Can you work these out from the model? Positions are in its coordinate system, mm. A direction names the side the tool comes from. Give positions to 0.01 mm unless a question says otherwise; leave off trailing zeros. Write each loop counter-clockwise with the first axis right and the second up, starting at its lowest first coordinate (ties: lowest second). Pieces come first, ordered by that corner, then holes. Notation, with made-up numbers: (-40, 35.5) -> (-34, 35.5) arc R26 ccw to (-34, 72.5) -> close; hole circle Ø1 at (68.25, 53). An arc over 180 degrees is marked (long way). One line per item, written item: value.
from build123d import *

# Parameters (mm, degrees)
FILLET1_R     = 1
CHAMFER1_SIZE = 0.5


with BuildPart() as part:
    # Sketch1 → Revolve1 (revolve)
    with BuildSketch(Plane.XY, mode=Mode.PRIVATE) as revolve1_sk:
        Polygon((-26, 0), (-25, 0), (-25, 8), (-13, 8), (-13, 0), (-15.5, 0), (-15.5, 2.5), (-22.5, 2.5), (-22.5, -1), (-26, -1), align=None)
    revolve(revolve1_sk.sketch.rotate(Axis((0, 0, 0), (0, 1, 0)), 270), axis=Axis((0, 0, 0), (0, 1, 0)))

    # Fillet1
    fillet1_edges = [part.edges().sort_by_distance(p)[0] for p in [
        (0, 8, 25),
        (0, 2.5, 22.5),
        (0, 2.5, 15.5),
    ]]
    fillet(fillet1_edges, radius=FILLET1_R)

    # Chamfer1
    chamfer1_edges = [part.edges().sort_by_distance(p)[0] for p in [
        (0, -1, 26),
        (0, -1, 22.5),
    ]]
    chamfer(chamfer1_edges, length=CHAMFER1_SIZE)


solid = part.part
1) For faces 1 (the face through (8.618, 0.486, -20.784)), 2 (the face through (-21, 0, 14)), 3 (the face through (7.91, 3.944, 10.316)), which set-ups out of +Z, -Z, +X, -X, +Y, -Y let a thin tool reach every point of the face, with its end or its side?
Answer list:
face 1: -Y
face 2: +Y
face 3: +Y, -Y
2) If we section it at C-C (y = 0.75): Write out the boundary of the cut face in (x, z).
Answer list:
outline: circle Ø50 at (0, 0); circle Ø31 at (0, 0); hole circle Ø45 at (0, 0); hole circle Ø26 at (0, 0)
3) If we section it at D-D (y = 3.5): Write out the boundary of the cut face in (x, z), and give its area (3 significant figures).
Answer list:
outline: circle Ø50 at (0, 0); hole circle Ø26 at (0, 0)
area: 1,430 mm^2
4) We'd pull the mould along X, two halves only. Please class faces 4 (the face through (16, 2.5, -5)), 5 (the face through (-7.509, 3.549, -23.846)), 6 (the face through (10, 8, -10)): released by +X, released by -X, zero draft, split by the parting line, or undercut.
Answer list:
face 4: undercut
face 5: split by the parting line
face 6: zero draft
5) I need wall thicknesses on L1, parallel to X at y = 0.45, z = 0; L2, parallel to Z at x = 10, y = 1.5; L3, parallel to X at y = 2.25, z = -11. Which ranges of each line are inside material? Lowest first, please.
Answer list:
L1: x = -25 to -22.5, -15.5 to -13, 13 to 15.5, 22.5 to 25
L2: z = -22.91 to -20.16, -11.84 to -8.31, 8.31 to 11.84, 20.16 to 22.91
L3: x = -22.45 to -19.24, -11.4 to -6.93, 6.93 to 11.4, 19.24 to 22.45
6) Will these pins go through, and if not, where does the flat tip stop? pin 1 (6 mm diameter, centred on x = 9.5, z = -0.5, fed in from -Y) (3 decimals); pin 2 (25 mm diameter, centred on x = -4.5, z = 2.5, fed in from -Y); pin 3 (5 mm diameter, centred on x = -3, y = 5.5, fed in from +Z) (3 decimals); pin 4 (4 mm diameter, centred on y = 3, z = 16, fed in from +X).
Answer list:
pin 1: passes through
pin 2: stops at y = 0
pin 3: stops at z = 24.995
pin 4: stops at x = 20.71
